Design review of the part shown in the three views and the two pictorial views. Dimensions are in mm from the part's minimum x, y and z. Round coordinates to 2 decimals unless told otherwise and drop trailing zeros. Order: outer loops, then holes, each group sorted by start corner. A loop starts at its lowest first (then second) coordinate and runs counter-clockwise, first axis right, second up. Notation, with made-up numbers: (-1.75, 26) - (37.25, 26) arc R24 cw to (37.25, 54) - close; hole circle Ø11 at (83, -12). An arc over 180 degrees is marked (long way). One line per item, written item: value.
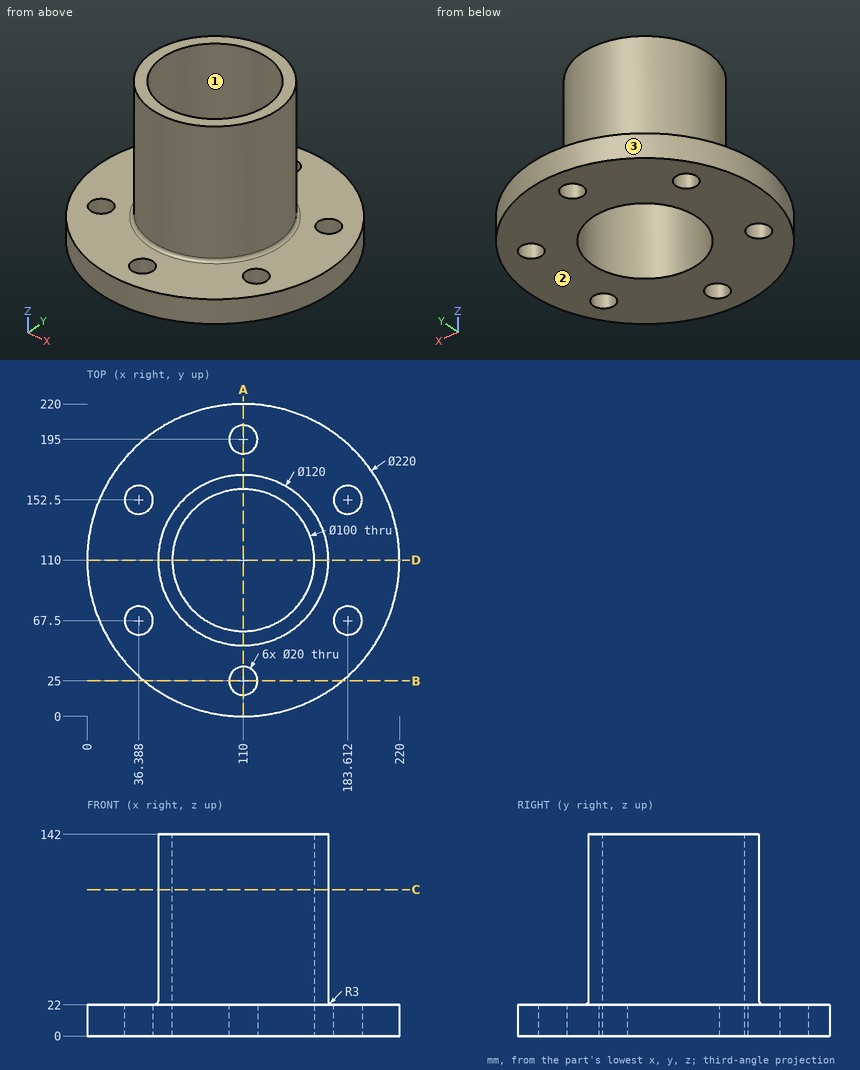
Item 1: The part is to be moulded in two halves that separate along Y. For the marked faces 1, 2 and 3, say which applies: +Y half, -Y half, draft (parallel to the pull), parting line (faces both ways), or undercut.
Returned:
face 1: undercut
face 2: draft
face 3: parting line
Item 2: Take a section at B-B (y = 25). Write out the cut boundary in (x, z).
Returned:
outline: (40.18, 0) - (100, 0) - (100, 22) - (40.18, 22) - close; (120, 0) - (179.82, 0) - (179.82, 22) - (120, 22) - close
Item 3: Wall thickness on line 1 (Y direction, x = 110, z = 60); line 2 (Z direction, x = 163, y = 22); line 3 (Y direction, x = 152, z = 62): over which ranges is each line inside the solid? List them lowest first.
Returned:
line 1: 50 to 60, 160 to 170
line 2: 0 to 22
line 3: 67.15 to 82.87, 137.13 to 152.85
Item 4: Take a section at A-A (x = 110). Write out the cut boundary in (y, z), plus the area to 3 significant figures.
Returned:
outline: (0, 0) - (15, 0) - (15, 22) - (0, 22) - close; (35, 0) - (60, 0) - (60, 142) - (50, 142) - (50, 25) arc R3 cw to (47, 22) - (35, 22) - close; (160, 0) - (185, 0) - (185, 22) - (173, 22) arc R3 cw to (170, 25) - (170, 142) - (160, 142) - close; (205, 0) - (220, 0) - (220, 22) - (205, 22) - close
area: 4,160 mm^2
Item 5: Take a section at D-D (y = 110). Write out the cut boundary in (x, z).
Returned:
outline: (0, 0) - (60, 0) - (60, 142) - (50, 142) - (50, 25) arc R3 cw to (47, 22) - (0, 22) - close; (160, 0) - (220, 0) - (220, 22) - (173, 22) arc R3 cw to (170, 25) - (170, 142) - (160, 142) - close
Item 6: Take a section at C-C (z = 103). Write out the cut boundary in (x, y).
Returned:
outline: circle Ø120 at (110, 110); hole circle Ø100 at (110, 110)
Item 7: For P1, Ø16, axis at x = 36.39, y = 67.5, coming from the -Z side; P2, Ø5, axis at x = 179.5, y = 52, coming from the +Z side; P3, Ø3, axis at x = 138, y = 165.5, coming from the +Z side; P4, Ø10, axis at y = 104, z = 65.5, coming from the -X side, all flat-tipped, find the tip position at first contact; note any pin that passes through.
Returned:
P1: through
P2: z = 22
P3: z = 23.12
P4: x = 50.01
